Part model, mm, in its own coordinate system. Face numbers are marked on the shaded views. Give positions to 0.01 mm unless a question says otherwise; leave off trailing zeros. Loops run counter-clockwise (first coordinate to the right, second up) from the corner with the lowest first, then second, coordinate; pieces in that order, holes last. Notation, with made-up numbers: M -16.75,53 L 38.25,53 A7 cw 38.25,60 Z; hole C 89,12 d1. An arc over 180 degrees is marked long. Answer in a Markdown table with one row per item.
from build123d import *

# Parameters (mm, degrees)
F0_W      = 100
F0_H      = 10
F0_W_2    = 63
F0_H_2    = 3
F1_DEPTH  = 4
F2_W      = 69
F2_H      = 10
F3_DEPTH  = 2
F4_R      = 2.5
F5_DEPTH  = 25
F6_R      = 2.5
F7_DEPTH  = 25
F8_W      = 9
F8_H      = 3
F9_DEPTH  = 2
F10_R     = 1.5
F11_DEPTH = 25


with BuildPart() as f1:
    # F0 (on Front) → F1 (new body)
    with BuildSketch(Plane.XZ):
        Rectangle(F0_W, F0_H)
        with Locations((0, -0.5)):
            Rectangle(F0_W_2, F0_H_2, mode=Mode.SUBTRACT)
    extrude(amount=F1_DEPTH)

    # F2 (on face) → F3 (cut)
    with BuildSketch(Plane.XZ.offset(4)):
        Rectangle(F2_W, F2_H)
    extrude(amount=-F3_DEPTH, mode=Mode.SUBTRACT)

    # F4 (on face) → F5 (cut)
    with BuildSketch(Plane.XZ.offset(4)):
        with Locations((-42.25, 0)):
            Circle(F4_R)
    extrude(amount=-F5_DEPTH, mode=Mode.SUBTRACT)

    # F6 (on face) → F7 (cut)
    with BuildSketch(Plane.XZ.offset(4)):
        with Locations((42.25, 0)):
            Circle(F6_R)
    extrude(amount=-F7_DEPTH, mode=Mode.SUBTRACT)

    # F8 (on face) → F9 (join)
    with BuildSketch(Plane(origin=(0, 0, 0), x_dir=(-1, 0, 0), z_dir=(0, 1, 0))):
        with Locations((27, -0.5)):
            Rectangle(F8_W, F8_H)
    extrude(amount=-F9_DEPTH)

    # F10 (on face) → F11 (cut)
    with BuildSketch(Plane(origin=(0, 0, 0), x_dir=(-1, 0, 0), z_dir=(0, 1, 0))):
        with Locations((27, -0.5)):
            Circle(F10_R)
    extrude(amount=-F11_DEPTH, mode=Mode.SUBTRACT)


solid = f1.part
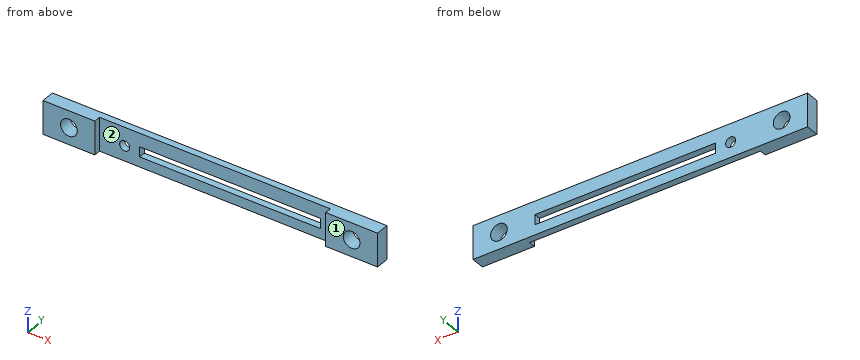
(1) Saw through at A-A (x = -42.25). Write the cut outline in (y, z), plus the area to 3 significant figures.
Recorded:
| item | result |
|---|---|
| outline | M -4,-5 L 0,-5 L 0,-2.5 L -4,-2.5 Z; M -4,2.5 L 0,2.5 L 0,5 L -4,5 Z |
| area | 20.0 mm^2 |
(2) Pin check, flat tip, straight feed: pin 1 Ø3.5 at (x, z) = (-27, -0.5) entering from -Y. Stop position of the tip, or through.
Recorded:
| item | result |
|---|---|
| pin 1 | stops at y = -2 |
(3) Pull direction X, two halves, no side cores. Call the marked faces 1 and 2: +X half, -X half, draft (parallel to the pull), parting line (faces both ways), or undercut.
Recorded:
| item | result |
|---|---|
| face 1 | draft |
| face 2 | undercut |
(4) Saw through at C-C (z = -4). Write the cut outline in (x, y).
Recorded:
| item | result |
|---|---|
| outline | M -50,-4 L -34.5,-4 L -34.5,-2 L 34.5,-2 L 34.5,-4 L 50,-4 L 50,0 L -50,0 Z |
(5) Saw through at D-D (x = -27). Write the cut outline in (y, z).
Recorded:
| item | result |
|---|---|
| outline | M -2,-5 L 0,-5 L 0,-2 L -2,-2 Z; M -2,1 L 0,1 L 0,5 L -2,5 Z |
(6) Saw through at B-B (y = -1.05). Write the cut outline in (x, z).
Recorded:
| item | result |
|---|---|
| outline | M -50,-5 L 50,-5 L 50,5 L -50,5 Z; hole C -42.25,0 d5; hole C -27,-0.5 d3; hole M -22.5,-2 L 31.5,-2 L 31.5,1 L -22.5,1 Z; hole C 42.25,0 d5 |
(7) Drill centre lines: line 1 along Z through (x, y) = (0, -0.55); line 2 along X through (y, z) = (-0.9, 1.25); line 3 along X through (y, z) = (-3.65, -4). Where is each one in solid material? Low to high.
Recorded:
| item | result |
|---|---|
| line 1 | z = -5 to -2, 1 to 5 |
| line 2 | x = -50 to -44.42, -40.08 to 40.08, 44.42 to 50 |
| line 3 | x = -50 to -34.5, 34.5 to 50 |
